Can you work these out from the model? Positions are in its coordinate system, mm. A direction names the side the tool comes from. Give positions to 0.01 mm unless a question says otherwise; leave off trailing zeros. Order: outer loops, then holes, each group sorted by start corner. A loop starts at its lowest first (then second) coordinate and runs counter-clockwise, first axis right, second up. Notation, with made-up numbers: M 18.25,6.5 L 36.25,6.5 A5 cw 36.25,10.5 Z; hole C 17.5,37.25 d10. An arc over 180 degrees is marked long. Answer as a JSON object with one key per item and string values.
```python
from build123d import *

# Parameters (mm, degrees)
SKETCH1_W           = 150
SKETCH1_H           = 80
SKETCH1_R           = 2.5
SKETCH1_R_2         = 1.5
SKETCH1_W_2         = 5
SKETCH1_H_2         = 20
BOSS_EXTRUDE1_DEPTH = 5


with BuildPart() as part:
    # Sketch1 → Boss-Extrude1 (new body)
    with BuildSketch(Plane.XY):
        with Locations((0, 10)):
            Rectangle(SKETCH1_W, SKETCH1_H)
        with Locations((-65, 43)):
            Circle(SKETCH1_R, mode=Mode.SUBTRACT)
        with Locations(Location((65, 43, 0), (0, 0, 180))):
            Circle(SKETCH1_R, mode=Mode.SUBTRACT)
        with Locations((65, -23)):
            Circle(SKETCH1_R, mode=Mode.SUBTRACT)
        with Locations(Location((-65, -23, 0), (0, 0, 180))):
            Circle(SKETCH1_R, mode=Mode.SUBTRACT)
        with Locations((-65, 30)):
            Circle(SKETCH1_R_2, mode=Mode.SUBTRACT)
        with Locations(Location((-65, -10, 0), (0, 0, 180))):
            Circle(SKETCH1_R_2, mode=Mode.SUBTRACT)
        with Locations((65, -10)):
            Circle(SKETCH1_R_2, mode=Mode.SUBTRACT)
        with Locations(Location((65, 30, 0), (0, 0, 180))):
            Circle(SKETCH1_R_2, mode=Mode.SUBTRACT)
        with Locations((-65, 10)):
            Rectangle(SKETCH1_W_2, SKETCH1_H_2, mode=Mode.SUBTRACT)
        with Locations((65, 10)):
            Rectangle(SKETCH1_W_2, SKETCH1_H_2, mode=Mode.SUBTRACT)
    extrude(amount=BOSS_EXTRUDE1_DEPTH)


solid = part.part
```
1) I want a section at C-C on x = 65. Write out the boundary of the cut face in (y, z), and give its area (3 significant figures).
Results found:
{"outline": "M -30,0 L -25.5,0 L -25.5,5 L -30,5 Z; M -20.5,0 L -11.5,0 L -11.5,5 L -20.5,5 Z; M -8.5,0 L 0,0 L 0,5 L -8.5,5 Z; M 20,0 L 28.5,0 L 28.5,5 L 20,5 Z; M 31.5,0 L 40.5,0 L 40.5,5 L 31.5,5 Z; M 45.5,0 L 50,0 L 50,5 L 45.5,5 Z", "area": "220 mm²"}
2) I want a section at D-D on y = -10. Write out the boundary of the cut face in (x, z).
Results found:
{"outline": "M -75,0 L -66.5,0 L -66.5,5 L -75,5 Z; M -63.5,0 L 63.5,0 L 63.5,5 L -63.5,5 Z; M 66.5,0 L 75,0 L 75,5 L 66.5,5 Z"}
3) I want a section at B-B on z = 1.85. Count the separate pieces of the cut face and the enclosed holes in it, and give its area (3 significant figures).
Results found:
{"separate pieces": "1", "enclosed holes": "10", "area": "11,700 mm²"}
4) Thinking about a two-plate mould opening in Y: for faces 1 (the face through (-65, 0, 2)), 2 (the face through (-1, 50, 2)), 3 (the face through (-75, 9, 2)), which applies, pulls with the +Y half, pulls with the -Y half, needs draft (parallel to the pull), parting line crosses it, or undercut?
Results found:
{"face 1": "undercut", "face 2": "pulls with the +Y half", "face 3": "needs draft"}
5) I need wall thicknesses on L1, parallel to X at y = -25, z = 3.7; L2, parallel to Y at x = 65, z = 1.7; L3, parallel to X at y = 12, z = 0.95. Which ranges of each line are inside material? Lowest first, please.
Results found:
{"L1": "x = -75 to -66.5, -63.5 to 63.5, 66.5 to 75", "L2": "y = -30 to -25.5, -20.5 to -11.5, -8.5 to 0, 20 to 28.5, 31.5 to 40.5, 45.5 to 50", "L3": "x = -75 to -67.5, -62.5 to 62.5, 67.5 to 75"}
6) I want a section at A-A on y = 8.5. Write out the boundary of the cut face in (x, z).
Results found:
{"outline": "M -75,0 L -67.5,0 L -67.5,5 L -75,5 Z; M -62.5,0 L 62.5,0 L 62.5,5 L -62.5,5 Z; M 67.5,0 L 75,0 L 75,5 L 67.5,5 Z"}
7) For faces 4 (the face through (65, 0, 2)), 5 (the face through (75, 9, 2)), which set-ups out of +Z, -Z, +X, -X, +Y, -Y let a thin tool reach every point of the face, with its end or its side?
Results found:
{"face 4": "+Z, -Z", "face 5": "+Z, -Z, +X, +Y, -Y"}
